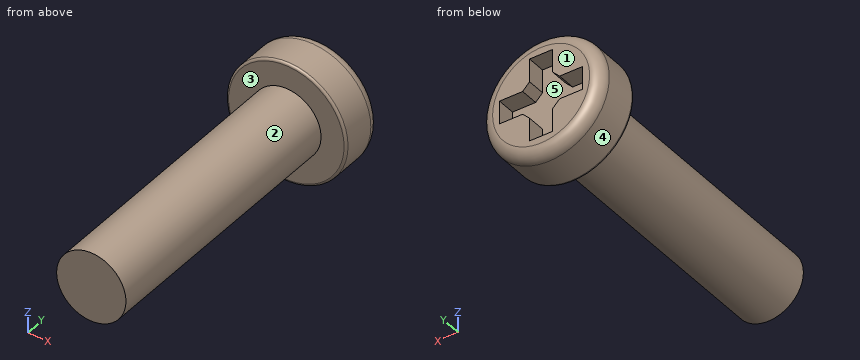
Autodesk Inventor part; units mm, degrees
ref_plane "YZ Plane" through (0, 0, 0) normal (1, 0, 0) x (0, 1, 0)
ref_plane "XZ Plane" through (0, 0, 0) normal (0, 1, 0) x (-1, 0, 0)
ref_plane "XY Plane" through (0, 0, 0) normal (0, 0, 1) x (1, 0, 0)
sketch "Sketch1" plane through (0, 0, 0) normal (0, 1, 0) x (-1, 0, 0)
  circle A0 centre (0, 0) radius 1.5
  dimension "d0" = 3
extrude "Extrusion1" add sketch "Sketch1" along normal blind 12
sketch "Sketch2" plane through (0, 12, 0) normal (0, 1, 0) x (1, 0, 0)
  circle A0 centre (0, 0) radius 2.6
  dimension "d3" = 5.2
extrude "Extrusion2" add sketch "Sketch2" along normal blind 2
sketch "Sketch3" plane through (0, 14, 0) normal (0, 1, 0) x (1, 0, 0)
  line L0 (-1.8, 0.5) -> (-0.8, 0.5)
  line L1 (-0.8, 0.5) -> (-0.5, 0.8)
  line L2 (-0.5, 0.8) -> (-0.5, 1.8)
  line L3 (-0.5, 1.8) -> (0.5, 1.8)
  line L4 (0.5, 1.8) -> (0.5, 0.8)
  line L5 (0.5, 0.8) -> (0.8, 0.5)
  line L6 (0.8, 0.5) -> (1.8, 0.5)
  line L7 (1.8, 0.5) -> (1.8, -0.5)
  line L8 (1.8, -0.5) -> (0.8, -0.5)
  line L9 (0.8, -0.5) -> (0.5, -0.8)
  line L10 (0.5, -0.8) -> (0.5, -1.8)
  line L11 (0.5, -1.8) -> (-0.5, -1.8)
  line L12 (-0.5, -1.8) -> (-0.5, -0.8)
  line L13 (-0.5, -0.8) -> (-0.8, -0.5)
  line L14 (-0.8, -0.5) -> (-1.8, -0.5)
  line L15 (-1.8, -0.5) -> (-1.8, 0.5)
  point P0 (0, 0)
  dimension "d6" = 1
  dimension "d7" = 1
  dimension "d8" = 1
  dimension "d9" = 1
  dimension "d11" = 1
  dimension "d12" = 1
  dimension "d13" = 1
  dimension "d14" = 1
  dimension "d15" = 1
  dimension "d16" = 1
  dimension "d17" = 135
  dimension "d18" = 135
  dimension "d19" = 135
  dimension "d20" = 0.5
  dimension "d21" = 0.5
  dimension "d22" = 1.8
  dimension "d23" = 1.8
  dimension "d24" = 0.5
extrude "Extrusion3" cut sketch "Sketch3" against normal blind 0.8
fillet "Fillet1" radius 0.5 1 edges at (-2.6, 14, 0)
fillet "Fillet2" radius 0.1 1 edges at (-2.6, 12, 0)
thread "Thread1"
equation "\"d7\" = d6"
equation "\"d8\" = d6"
equation "\"d9\" = d6"
equation "\"d11\" = d6"
equation "\"d12\" = d6"
equation "\"d13\" = d6"
equation "\"d14\" = d6"
equation "\"d15\" = d6"
equation "\"d16\" = d6"
equation "\"d18\" = d17"
equation "\"d19\" = d17"
properties part number "plastic_screw_3_x_12"
Work out the finished part from the listing and answer in its coordinate system (mm). Face numbers are marked on the shaded views. A direction names the side the tool comes from. Give positions to 0.01 mm unless a question says otherwise; leave off trailing zeros. Order: outer loops, then holes, each group sorted by start corner. A loop starts at its lowest first (then second) coordinate and runs counter-clockwise, first axis right, second up. Notation, with made-up numbers: (53.25, 11.25) -> (104.25, 11.25) arc R26 ccw to (104.25, 50.25) -> close; hole circle Ø9 at (16.25, -2.5). An arc over 180 degrees is marked (long way). One line per item, written item: value.
Item 1: Find section C-C, the plane y = 2. Give the vertices of the cut face in (x, z).
Answer sheet:
outline: circle Ø3 at (0, 0)
Item 2: Find section B-B, the plane x = 0. Give the vertices of the cut face in (y, z), plus the area to 3 significant figures.
Answer sheet:
outline: (0, -1.5) -> (12, -1.5) -> (12, -2.5) arc R0.1 ccw to (12.1, -2.6) -> (13.5, -2.6) arc R0.5 ccw to (14, -2.1) -> (14, -1.8) -> (13.2, -1.8) -> (13.2, 1.8) -> (14, 1.8) -> (14, 2.1) arc R0.5 ccw to (13.5, 2.6) -> (12.1, 2.6) arc R0.1 ccw to (12, 2.5) -> (12, 1.5) -> (0, 1.5) -> close
area: 43.4 mm²
Item 3: Find section A-A, the plane z = 0. Give the vertices of the cut face in (x, y), plus the area to 3 significant figures.
Answer sheet:
outline: (-2.6, 12.1) arc R0.1 ccw to (-2.5, 12) -> (-1.5, 12) -> (-1.5, 0) -> (1.5, 0) -> (1.5, 12) -> (2.5, 12) arc R0.1 ccw to (2.6, 12.1) -> (2.6, 13.5) arc R0.5 ccw to (2.1, 14) -> (1.8, 14) -> (1.8, 13.2) -> (-1.8, 13.2) -> (-1.8, 14) -> (-2.1, 14) arc R0.5 ccw to (-2.6, 13.5) -> close
area: 43.4 mm²
Item 4: Determine the mould class of the marked faces 3, 4 and 5 for opening direction X: released by +X, released by -X, zero draft, split by the parting line, or undercut.
Answer sheet:
face 3: zero draft
face 4: split by the parting line
face 5: undercut
Item 5: A tool of negligible diameter and unlimited length cuts with its end or side. For the marked faces 1 and 2, from which of +Z, -Z, +X, -X, +Y, -Y can it reach the whole face along a straight path? Write none if from no direction.
Answer sheet:
face 1: +Z, -Z, +X, -X, +Y
face 2: -Y
Item 6: Straight lines are drawn through the part: probe 1 along Y at (x, z) = (-0.4, 2.05); probe 2 along Y at (x, z) = (0.4, -0.95); probe 3 along Z at (x, y) = (0.3, 13.25). For each, find the intervals that lie inside material, in ascending order.
Answer sheet:
probe 1: 12 to 14
probe 2: 0 to 13.2
probe 3: -2.58 to -1.8, 1.8 to 2.58
Item 7: Flat-ended cylindrical pins translate along their axes: P1, Ø0.6, axis at x = 1.5, y = 13.5, coming from the +Z side; P2, Ø0.9, axis at y = 14, z = -1.5, coming from the -X side; P3, Ø0.6, axis at y = 13.5, z = -1, coming from the +X side. Find the tip coordinate at first contact, or state that the pin passes through.
Answer sheet:
P1: z = 2.31
P2: x = -2.28
P3: x = 2.5
